from build123d import *

# Parameters (mm, degrees)
F0_R             = 30
F0_R_2           = 1.5
F1_DEPTH         = 2
F2_R             = 7.5
F2_R_2           = 1.5
F3_DEPTH         = 2
F4_R             = 3
F4_R_2           = 1.5
F5_DEPTH         = 3
F6_SIZE          = 1
F7_R             = 30
F7_R_2           = 4
F8_DEPTH         = 5
F10_DEPTH        = 25
F10_COPIES_COUNT = 4
F11_R            = 3


# Not quite as in the source:
# - a pattern or mirror of a feature is missing from the dataset's text; its kind, count and spacing are read off the source's solid


with BuildPart() as f1:
    # F0 (on Top) → F1 (new body)
    with BuildSketch(Plane.XY):
        Circle(F0_R)
        Circle(F0_R_2, mode=Mode.SUBTRACT)
    extrude(amount=F1_DEPTH)

    # F2 (on face) → F3 (join)
    with BuildSketch(Plane.XY.offset(2)):
        Circle(F2_R)
        Circle(F2_R_2, mode=Mode.SUBTRACT)
    extrude(amount=F3_DEPTH)

    # F4 (on face) → F5 (cut)
    with BuildSketch(Plane.XY.offset(4)):
        Circle(F4_R)
        Circle(F4_R_2, mode=Mode.SUBTRACT)
    extrude(amount=-F5_DEPTH, mode=Mode.SUBTRACT)

    # F6
    f6_edges = [f1.edges().sort_by_distance(p)[0] for p in [
        (-7.5, 0, 4),
    ]]
    chamfer(f6_edges, length=F6_SIZE)

    # F7 (on face) → F8 (join)
    with BuildSketch(Plane(origin=(0, 0, 0), x_dir=(1, 0, 0), z_dir=(0, 0, -1))):
        Circle(F7_R)
        Circle(F7_R_2, mode=Mode.SUBTRACT)
    extrude(amount=F8_DEPTH)

    # F9 (on face) → F10 (cut)
    with BuildSketch(Plane.XY.offset(2)):
        with BuildLine():
            Line((2, -8.7749643874), (2, -25.9229627936))
            ThreePointArc((2, -25.9229627936), (18.3847763109, -18.3847763109), (25.9229627936, -2))
            Line((25.9229627936, -2), (8.7749643874, -2))
            ThreePointArc((8.7749643874, -2), (6.3639610307, -6.3639610307), (2, -8.7749643874))
        make_face()
    f10 = extrude(amount=-F10_DEPTH, mode=Mode.SUBTRACT)

    # F10_copies: F10 ×4 about axis
    f10_copies_axis = Axis((0, 0, 0), (0, 0, 1))
    for i in range(1, F10_COPIES_COUNT):
        add(f10.rotate(f10_copies_axis, i * 360 / F10_COPIES_COUNT), mode=Mode.SUBTRACT)

    # F11
    f11_edges = [f1.edges().sort_by_distance(p)[0] for p in [
        (8.774964, -2, -1.5),
        (2, -25.922963, -1.5),
        (25.922963, -2, -1.5),
        (2, -8.774964, -1.5),
        (-2, -8.774964, -1.5),
        (-2, -25.922963, -1.5),
        (-8.774964, -2, -1.5),
        (-25.922963, -2, -1.5),
        (-8.774964, 2, -1.5),
        (-25.922963, 2, -1.5),
        (-2, 25.922963, -1.5),
        (-2, 8.774964, -1.5),
        (2, 8.774964, -1.5),
        (2, 25.922963, -1.5),
        (25.922963, 2, -1.5),
        (8.774964, 2, -1.5),
    ]]
    fillet(f11_edges, radius=F11_R)

    # F12 (on Front) → F13 (revolve)
    with BuildSketch(Plane.XZ):
        with BuildLine():
            Line((31.1325030024, 2), (30, 2))
            Line((30, 2), (30, -5))
            Line((30, -5), (31.1325030024, -5))
            ThreePointArc((31.1325030024, -5), (30.5, -1.5), (31.1325030024, 2))
        make_face()
    revolve(axis=Axis((0, 0, 4), (0, 0, 1)))


solid = f1.part
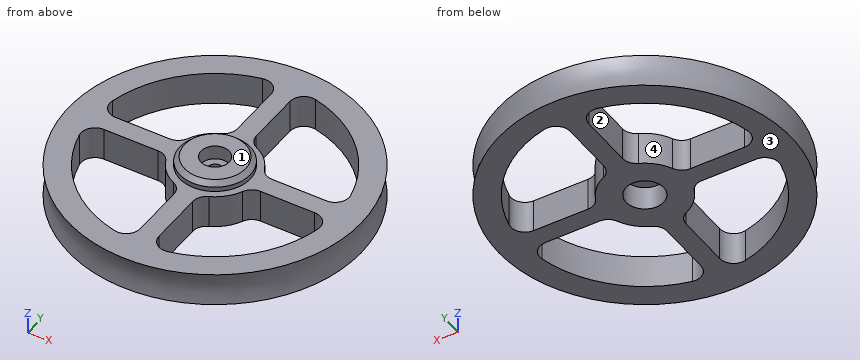
Source: CAD feature listing. Evaluate the final solid. Frame: model axes, mm. Face numbers are marked on the shaded views. A direction names the side the tool comes from. Give positions to 0.01 mm unless a question says otherwise; leave off trailing zeros. Order: outer loops, then holes, each group sorted by start corner. A loop starts at its lowest first (then second) coordinate and runs counter-clockwise, first axis right, second up. Notation, with made-up numbers: (67, 21) -> (85, 21) arc R23 ccw to (85, 54) -> close; hole circle Ø6 at (84, -25.75). An arc over 180 degrees is marked (long way). Write item = value, one per line.
Item 1: Contact query for flat-ended pins moving along their axis: pin 1 (7 mm diameter, centred on x = 0, y = 0, fed in from -Z); pin 2 (3.5 mm diameter, centred on x = -17.5, z = -2.5, fed in from -Y); pin 3 (4 mm diameter, centred on y = -20.5, z = -3, fed in from -X); pin 4 (6.5 mm diameter, centred on x = -1, y = -0.5, fed in from -Z). Output: stop coordinate, or through.
Check result:
pin_1 = 0
pin_2 = -26.21
pin_3 = -24.46
pin_4 = -5
Item 2: Section query C-C (z = -2). State how many separate pieces and enclosed holes the cut face has, then the cut area to 3 significant figures.
Check result:
separate_pieces = 1
enclosed_holes = 5
area = 1,310 mm²
Item 3: Section query A-A (x = 0). Output: boundary loops of the cut face in (y, z).
Check result:
outline = (-31.13, -5) -> (-4, -5) -> (-4, 0) -> (-1.5, 0) -> (-1.5, 1) -> (-3, 1) -> (-3, 4) -> (-6.5, 4) -> (-7.5, 3) -> (-7.5, 2) -> (-31.13, 2) arc R10 cw to start; (1.5, 0) -> (4, 0) -> (4, -5) -> (31.13, -5) arc R10 cw to (31.13, 2) -> (7.5, 2) -> (7.5, 3) -> (6.5, 4) -> (3, 4) -> (3, 1) -> (1.5, 1) -> close
Item 4: Mould query, pull axis X, two halves, no side actions, for the marked faces 1 and 2. Classes: +X half, -X half, draft (parallel to the pull), parting line (faces both ways), or undercut.
Check result:
face_1 = draft
face_2 = undercut
Item 5: Set-up query: the marked faces 3 and 4. Return all of +Z, -Z, +X, -X, +Y, -Y with unobstructed straight access to the full face (end or side cutting, diameter ignored); none if empty.
Check result:
face_3 = -Z, +X, -X, +Y, -Y
face_4 = +Z, -Z
Item 6: Ray query, probe 1 along X at (y, z) = (-19, -0.5); probe 2 along X at (y, z) = (-12, 1); probe 3 along Y at (x, z) = (7, -1.5). Return the intervals inside material, ascending.
Check result:
probe_1 = -23.92 to -17.75, -2 to 2, 17.75 to 23.92
probe_2 = -28.39 to -23.07, -2 to 2, 23.07 to 28.39
probe_3 = -29.69 to -25.04, -5.66 to 5.66, 25.04 to 29.69
